```python
from build123d import *

# Parameters (mm, degrees)
RESSALTO_EXTRUS_O2_START         = -0.25
ESBO_O2_W                        = 6.85008846
ESBO_O2_H                        = 25
RESSALTO_EXTRUS_O2_DEPTH         = 3.55
ESBO_O3_W                        = 39.35008846
ESBO_O3_H                        = 25
RESSALTO_EXTRUS_O3_DEPTH         = 3
ESBO_O4_W                        = 9.35
ESBO_O4_H                        = 25
RESSALTO_EXTRUS_O4_DEPTH         = 3
CBORE_FOR_M2_5_SHCS2_D           = 2.9
CBORE_FOR_M2_5_SHCS2_DEPTH       = 3
CBORE_FOR_M2_5_SHCS2_CBORE_D     = 5.5
CBORE_FOR_M2_5_SHCS2_CBORE_DEPTH = 2
CBORE_FOR_M2_5_SHCS2_TIP         = 0.871247898
CBORE_FOR_M2_5_SHCS3_D           = 2.9
CBORE_FOR_M2_5_SHCS3_CBORE_D     = 5.5
CBORE_FOR_M2_5_SHCS3_CBORE_DEPTH = 5


with BuildPart() as part:
    # Esboço2 → Ressalto-extrusão2 (new body)
    with BuildSketch(Plane.XY.offset(RESSALTO_EXTRUS_O2_START)):
        with Locations((1.92504423, -10)):
            Rectangle(ESBO_O2_W, ESBO_O2_H)
    extrude(amount=-RESSALTO_EXTRUS_O2_DEPTH)

    # Esboço3 → Ressalto-extrusão3 (add)
    with BuildSketch(Plane(origin=(0, 0, -3.8), x_dir=(-1, 0, 0), z_dir=(0, 0, -1))):
        with Locations((14.32495577, -10)):
            Rectangle(ESBO_O3_W, ESBO_O3_H)
    extrude(amount=RESSALTO_EXTRUS_O3_DEPTH)

    # Esboço4 → Ressalto-extrusão4 (add)
    with BuildSketch(Plane.ZY.offset(34)):
        with Locations((-2.125, -10)):
            Rectangle(ESBO_O4_W, ESBO_O4_H)
    extrude(amount=RESSALTO_EXTRUS_O4_DEPTH)

    # CBORE for M2.5 SHCS2
    with Locations(Plane(origin=(-37, -1.5, 0), x_dir=(0, 0, -1), z_dir=(-1, 0, 0))):
        with Locations((0, 0), (0, 17)):
            CounterBoreHole(CBORE_FOR_M2_5_SHCS2_D / 2, CBORE_FOR_M2_5_SHCS2_CBORE_D / 2, CBORE_FOR_M2_5_SHCS2_CBORE_DEPTH, depth=CBORE_FOR_M2_5_SHCS2_DEPTH)
            with Locations((0, 0, -(CBORE_FOR_M2_5_SHCS2_DEPTH + CBORE_FOR_M2_5_SHCS2_TIP / 2))):  # 118° drill point
                Cone(0, CBORE_FOR_M2_5_SHCS2_D / 2, CBORE_FOR_M2_5_SHCS2_TIP, mode=Mode.SUBTRACT)

    # CBORE for M2.5 SHCS3 (through all)
    with Locations(Plane(origin=(0, 0, -6.8), x_dir=(-1, 0, 0), z_dir=(0, 0, -1))):
        with Locations((-2.8, -1.5), (-2.8, -18.5)):
            CounterBoreHole(CBORE_FOR_M2_5_SHCS3_D / 2, CBORE_FOR_M2_5_SHCS3_CBORE_D / 2, CBORE_FOR_M2_5_SHCS3_CBORE_DEPTH)


solid = part.part
```
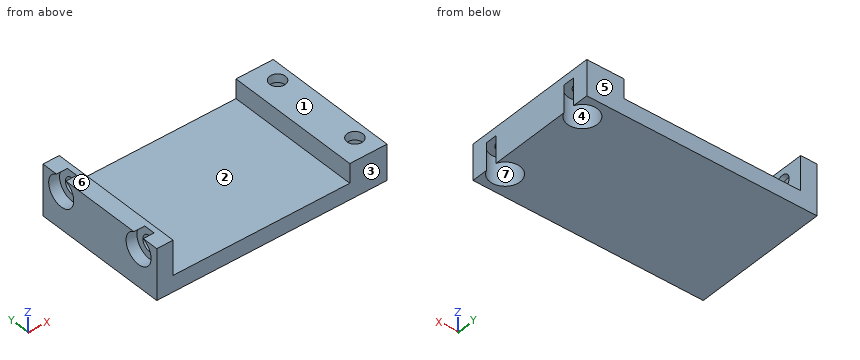
For this review, take the finished solid that the model builds, in its own axes (mm). Face numbers are marked on the shaded views. A direction names the side the tool comes from. Round coordinates to 2 decimals unless told otherwise and drop trailing zeros. Write each loop counter-clockwise with the first axis right and the second up, starting at its lowest first coordinate (ties: lowest second). Pieces come first, ordered by that corner, then holes. Notation, with made-up numbers: M -27.5,1.25 L 13.5,1.25 A32 ccw 13.5,39.25 Z; hole C 3.5,71.25 d7. An arc over 180 degrees is marked long. One line per item, written item: value. Start each with the question number.
(1) Wall thickness on line 1 (Y direction, x = 2.8, z = -3.55); line 2 (Y direction, x = -34.6, z = 0); line 3 (X direction, y = -14, z = -3): over which ranges is each line inside the solid? List them lowest first.
(2) We need section D-D (x = -26). Give the boundary of the cut face in (y, z), and give its area (3 significant figures).
(3) Machinability: for the marked faces 1, 2 and 3, which of the approach directions +Z, -Z, +X, -X, +Y, -Y give a long, thin tool a straight path to every point of the face, cutting with its end or side? Answer none if there is none.
(4) We need section A-A (y = -1.5). Give the boundary of the cut face in (x, z), and give its area (3 significant figures).
(5) We need section C-C (y = -8.5). Give the boundary of the cut face in (x, z), and give its area (3 significant figures).
(6) We need section B-B (x = 2.8). Give the boundary of the cut face in (y, z), and give its area (3 significant figures).
(7) Insertion check: pin 1 (4 mm diameter, centred on x = 2.5, y = -1, fed in from -Z); pin 2 (9 mm diameter, centred on x = 2.8, y = -1.5, fed in from +Z); pin 3 (1.5 mm diameter, centred on y = -0.5, z = 1, fed in from -X); pin 4 (2.5 mm diameter, centred on x = 2.8, y = -1.5, fed in from -Z). Each pin has a flat end and moves straight along its axis. Give the tip position at first contact, or say it passes through.
(8) The part is to be moulded in two halves that separate along Y. For the marked faces 4, 5, 6 and 7, say which applies: released by +Y, released by -Y, zero draft, split by the parting line, or undercut.
Result:
1. line 1: -22.5 to -21.25, -15.75 to -4.25, 1.25 to 2.5
1. line 2: -22.5 to -19.95, -17.05 to -2.95, -0.05 to 2.5
1. line 3: -37 to -34, -1.5 to 5.35
2. outline: M -22.5,-6.8 L 2.5,-6.8 L 2.5,-3.8 L -22.5,-3.8 Z
2. area: 75.0 mm²
3. face 1: +Z, +X, +Y, -Y
3. face 2: +Z, +Y, -Y
3. face 3: +Z, -Z, +X, -X, -Y
4. outline: M -37,-6.8 L 0.05,-6.8 L 0.05,-1.8 L 1.35,-1.8 L 1.35,-0.25 L -1.5,-0.25 L -1.5,-3.8 L -34,-3.8 L -34,-1.45 L -35,-1.45 L -35,-2.75 L -37,-2.75 Z; M -35,1.45 L -34,1.45 L -34,2.55 L -35,2.55 Z; M 4.25,-1.8 L 5.35,-1.8 L 5.35,-0.25 L 4.25,-0.25 Z
4. area: 126 mm²
5. outline: M -37,-6.8 L 5.35,-6.8 L 5.35,-0.25 L -1.5,-0.25 L -1.5,-3.8 L -34,-3.8 L -34,2.55 L -37,2.55 Z
5. area: 170 mm²
6. outline: M -22.5,-6.8 L -21.25,-6.8 L -21.25,-1.8 L -19.95,-1.8 L -19.95,-0.25 L -22.5,-0.25 Z; M -17.05,-1.8 L -15.75,-1.8 L -15.75,-6.8 L -4.25,-6.8 L -4.25,-1.8 L -2.95,-1.8 L -2.95,-0.25 L -17.05,-0.25 Z; M -0.05,-1.8 L 1.25,-1.8 L 1.25,-6.8 L 2.5,-6.8 L 2.5,-0.25 L -0.05,-0.25 Z
6. area: 99.8 mm²
7. pin 1: z = -1.8
7. pin 2: z = -0.25
7. pin 3: x = -35
7. pin 4: through
8. face 4: undercut
8. face 5: released by +Y
8. face 6: zero draft
8. face 7: undercut
